```python
from build123d import *

# Parameters (mm, degrees)
F0_R     = 101.6
F1_DEPTH = 25.4
F3_D     = 12.7
F4_R     = 6.35
F5_DEPTH = 127


with BuildPart() as f1:
    # F0 (on Top) → F1 (new body)
    with BuildSketch(Plane.XY):
        Circle(F0_R)
    extrude(amount=F1_DEPTH)

    # F3 (through all)
    with Locations(Plane(origin=(0, 0, 0), x_dir=(1, 0, 0), z_dir=(0, 0, -1))):
        with Locations((0, -88.9)):
            Hole(F3_D / 2)

    # F4 (on face) → F5 (join)
    with BuildSketch(Plane.XY.offset(25.4)):
        with Locations((-72.815311, 0)):
            Circle(F4_R)
    extrude(amount=F5_DEPTH)


solid = f1.part
```
Model file for the job. Use its own axes, mm. A direction names the side the tool comes from. Round coordinates to 2 decimals unless told otherwise and drop trailing zeros. Write each loop counter-clockwise with the first axis right and the second up, starting at its lowest first coordinate (ties: lowest second). Pieces come first, ordered by that corner, then holes. Notation, with made-up numbers: M 85,40 L 121,40 A12 cw 121,52 Z; hole C 50,53.25 d4. An arc over 180 degrees is marked long. Put each result on its own line as item: value.
Item 1: Tool access for faces 4 (the cylindrical face through (-79.16, 0.28, 88.01)), 5 (the flat face through (-1, 1, 0)): list every direction of +Z, -Z, +X, -X, +Y, -Y with a clear straight run to the whole face (end or side of a thin tool).
Responses:
face 4: +Z
face 5: -Z, +X, -X, +Y, -Y
Item 2: Mould opens along X. For faces 1 (the cylindrical face through (-22.025, -99.184, 12.522)), 2 (the cylindrical face through (0.8, 82.6, 12.9)), 3 (the flat face through (-73, 0, 152.4)) say: +X half, -X half, draft (parallel to the pull), parting line (faces both ways), or undercut.
Responses:
face 1: parting line
face 2: undercut
face 3: draft
Item 3: Cut at C-C (z = 20.5). List the corners of the cut face in (x, y).
Responses:
outline: C 0,0 d203.2; hole C 0,88.9 d12.7
Item 4: Flat gauge pins, fed straight in: P1, Ø3, axis at y = 4.5, z = 96.5, coming from the +X side; P2, Ø6, axis at x = -71.5, z = 19, coming from the -Y side. Where does each tip first touch, or does it go through?
Responses:
P1: x = -67.22
P2: y = -75.04
Item 5: Cut at B-B (y = 0). List the corners of the cut face in (x, z).
Responses:
outline: M -101.6,0 L 101.6,0 L 101.6,25.4 L -66.47,25.4 L -66.47,152.4 L -79.17,152.4 L -79.17,25.4 L -101.6,25.4 Z
Item 6: Cut at D-D (y = 88.9). List the corners of the cut face in (x, z), and give its area (3 significant figures).
Responses:
outline: M -49.19,0 L -6.35,0 L -6.35,25.4 L -49.19,25.4 Z; M 6.35,0 L 49.19,0 L 49.19,25.4 L 6.35,25.4 Z
area: 2,180 mm²
Item 7: Cut at A-A (x = 0). List the corners of the cut face in (y, z).
Responses:
outline: M -101.6,0 L 82.55,0 L 82.55,25.4 L -101.6,25.4 Z; M 95.25,0 L 101.6,0 L 101.6,25.4 L 95.25,25.4 Z
Item 8: Probe L1, parallel to Y at x = 0, z = 11; L2, parallel to Z at x = -46, y = 56.5; L3, parallel to X at y = 88.9, z = 16. List the from-to ranges inside material, lowest first. Write a range as from..to.
Responses:
L1: -101.6..82.55, 95.25..101.6
L2: 0..25.4
L3: -49.19..-6.35, 6.35..49.19
